Geometry check sheet. Reference: the model listing, model coordinates, mm. A direction names the side the tool comes from. Round coordinates to 2 decimals unless told otherwise and drop trailing zeros. Write each loop counter-clockwise with the first axis right and the second up, starting at its lowest first coordinate (ties: lowest second). Pieces come first, ordered by that corner, then holes. Notation, with made-up numbers: M 8,-1 L 61,-1 A21 ccw 61,4 Z; hole C -16,-30 d10. An arc over 180 degrees is marked long. Answer in a Markdown table with one row per item. Add a question column.
from build123d import *

# Parameters (mm, degrees)
F1_DEPTH = 2.794
F2_R     = 3.81
F3_DEPTH = 2.794
F4_R     = 3.175
F5_DEPTH = 5.08
F6_R     = 3.5648567011
F7_DEPTH = 1.27
F8_R     = 3.2240766962
F9_DEPTH = 7.62
F9_TAPER = 8


with BuildPart() as f1:
    # F0 (on Front) → F1 (new body)
    with BuildSketch(Plane.XZ):
        Polygon((3.96875, -2.2913588808), (3.96875, 2.2913588808), (0, 4.5827177617), (-3.96875, 2.2913588808), (-3.96875, -2.2913588808), (0, -4.5827177617), align=None)
    extrude(amount=F1_DEPTH)

    # F2 (on face) → F3 (join)
    with BuildSketch(Plane.XZ.offset(2.794)):
        Circle(F2_R)
    extrude(amount=F3_DEPTH)

    # F4 (on face) → F5 (join)
    with BuildSketch(Plane.XZ.offset(5.588)):
        Circle(F4_R)
    extrude(amount=F5_DEPTH)

    # F6 (on face) → F7 (join)
    with BuildSketch(Plane(origin=(0, 0, 0), x_dir=(-1, 0, 0), z_dir=(0, 1, 0))):
        Circle(F6_R)
    extrude(amount=F7_DEPTH)

    # F8 (on face) → F9 (join)
    with BuildSketch(Plane(origin=(0, 1.27, 0), x_dir=(-1, 0, 0), z_dir=(0, 1, 0))):
        Circle(F8_R)
    extrude(amount=F9_DEPTH, taper=F9_TAPER)


solid = f1.part
Item 1: Access from +Z, -Z, +X, -X, +Y, -Y to the whole of each face (thin tool, end or side, straight path). Record for faces 1 (the cylindrical face through (0.464, 0.626, 3.535)), 2 (the flat face through (-1.96, -1.38, 3.45)), 3 (the cylindrical face through (-0.83, -4.17, -3.72)).
Item 2: Scan lines: probe 1 along X at (y, z) = (-2.75, -2.75); probe 2 along Z at (x, y) = (0, -8.5) (3 decimals); probe 3 along Y at (x, z) = (-2, 3). Record each from-to range of solid material in increasing order. Write a range as from..to.
Item 3: Gauge pin test, flat ends, axial feed: pin 1 Ø5 at (y, z) = (-4, 3) entering from -X; pin 2 Ø5 at (y, z) = (5.5, -1) entering from -X; pin 3 Ø4 at (y, z) = (-5, -0.5) entering from +X. Record the tip position at first contact, or that the pin passes through.
Item 4: Section check B-B, the plane y = 6.5. Record the boundary of the cut face in (x, z).
Item 5: Section check A-A, the plane y = -6.5. Record the boundary of the cut face in (x, z) (3 decimals), and give its area (3 significant figures).
Result sheet:
| question | item | result |
|---|---|---|
| 1 | face 1 | +Y |
| 1 | face 2 | +Z, -X, +Y, -Y |
| 1 | face 3 | -Y |
| 2 | probe 1 | x = -3.17..3.17 |
| 2 | probe 2 | z = -3.175..3.175 |
| 2 | probe 3 | y = -5.59..0 |
| 3 | pin 1 | stops at x = -3.97 |
| 3 | pin 2 | stops at x = -2.96 |
| 3 | pin 3 | stops at x = 3.81 |
| 4 | outline | C 0,0 d4.98 |
| 5 | outline | C 0,0 d6.35 |
| 5 | area | 31.7 mm^2 |
